Autodesk Inventor part; units mm, degrees
ref_plane "YZ Plane" through (0, 0, 0) normal (1, 0, 0) x (0, 1, 0)
ref_plane "XZ Plane" through (0, 0, 0) normal (0, 1, 0) x (-1, 0, 0)
ref_plane "XY Plane" through (0, 0, 0) normal (0, 0, 1) x (1, 0, 0)
sketch "Sketch1" plane through (0, 0, 0) normal (0, 0, 1) x (1, 0, 0)
  circle A0 centre (0, 0) radius 195 construction
  line L0 (0, 195) -> (0, 225) construction
  line L1 (0, 195) -> (0, 165) construction
  circle A1 centre (0, 0) radius 165
  circle A2 centre (0, 0) radius 225
  line L2 (-165, 0) -> (-165, 80)
  line L3 (-165, 80) -> (-225, 80)
  line L4 (-225, 80) -> (-225, 0)
  line L5 (165, 0) -> (165, 80)
  line L6 (165, 80) -> (225, 80)
  line L7 (225, 80) -> (225, 0)
  line L8 (-225, 0) -> (-165, 0)
  line L9 (165, 0) -> (225, 0)
  line L10 (-225, 0) -> (-285, 0)
  line L11 (-285, 0) -> (-285, -50)
  line L12 (-285, -50) -> (-219.3741, -50)
  line L13 (225, 0) -> (285, 0)
  line L14 (285, 0) -> (285, -50)
  line L15 (285, -50) -> (219.3741, -50)
  dimension "d13" = 390
  dimension "d26" = 80
  dimension "d36" = 60
  dimension "d40" = 60
  dimension "d41" = 50
extrude "Extrusion1" add sketch "Sketch1" against normal blind 30 contours L9 A2 L8 A1 | L13 L14 L15 A2 | A2 L12 L11 L10
sketch "Sketch4" plane through (0, 0, 0) normal (0, 0, 1) x (1, 0, 0)
  circle A0 centre (38.0426, -191.2531) radius 6.5
  line L0 (0, 0) -> (38.0426, -191.2531) construction
  line L1 (0, 0) -> (0, -276.8337) construction
  dimension "d17" = 13
  dimension "d27" = 195
  dimension "d35" = 11.25
extrude "Extrusion4" cut sketch "Sketch4" against normal through all
sketch "Sketch5" plane through (0, 0, 0) normal (0, 0, 1) x (1, 0, 0)
  circle A0 centre (38.0426, -191.2531) radius 6.5
  circle A1 centre (38.0426, -191.2531) radius 17.5
  point P0 (0, 0)
  dimension "d23" = 35
extrude "Extrusion5" cut sketch "Sketch5" against normal blind 15
pattern_circular "Circular Pattern3" count 8 over 157.5 about axis through (0, 0, 0) along (0, 0, -1) of "Extrusion4", "Extrusion5" both ways yes
sketch "Sketch7" plane through (-285, 0, 0) normal (0, 1, 0) x (1, 0, 0)
  circle A0 centre (25, 15) radius 7
  line L0 (0, 0) -> (0, 30)
  point P0 (285, 0)
  point P1 (0, 15)
  dimension "d42" = 14
  dimension "d43" = 25
extrude "Extrusion7" cut sketch "Sketch7" against normal through all
mirror "Mirror1" about plane through (0, 0, 0) normal (1, 0, 0) of "Extrusion7"
equation "\"d13\" = Шпил_пласт_НОС_диам_центров"
equation "\"d40\" = d36"
equation "\"d27\" = 0.5 * Шпил_пласт_НОС_диам_центров"
equation "\"BendReliefDepth\" = 0.5 * Thickness"
properties part number "ДМФ 091 Постель НОС"
Geometry: final body of the model. Coordinates: model frame, mm. A direction names the side the tool comes from. Coordinates: 2 decimals unless noted, no trailing zeros. Order: outer loops, then holes, each group sorted by start corner. A loop starts at its lowest first (then second) coordinate and runs counter-clockwise, first axis right, second up. Notation, with made-up numbers: (58.5, -5) - (78.5, -5) arc R16 cw to (78.5, 11) - close; hole circle Ø3 at (69.25, 4.25). An arc over 180 degrees is marked (long way). Return JSON: item names as keys, results as strings. Group by question number.
1. Cut plane B-B (y = -76). Output: boundary loops of the cut face in (x, z).
2. Cut plane C-C (x = 0). Output: boundary loops of the cut face in (y, z).
3. Cut plane D-D (x = -234.5). Output: boundary loops of the cut face in (y, z).
4. Pull-direction query (Y, two-part tool) for faces 3 (the face through (46, -191, -15)), 4 (the face through (252.6, -50, -14.8)), 5 (the face through (41.04, -197.02, -22.4)), 6 (the face through (-22, -170, -30)); classes: pulls with the +Y half, pulls with the -Y half, needs draft (parallel to the pull), parting line crosses it, or undercut.
5. Pin query (flat end, axial travel): pin 1 (10.5 mm diameter, centred on x = 167, y = -117, fed in from +Z); pin 2 (12 mm diameter, centred on x = 185, z = -9.5, fed in from -Y); pin 3 (1 mm diameter, centred on x = 50, z = -7, fed in from -Y). Return the tip coordinate at first contact, or that it passes through.
6. Material intervals for line 1 along X through (y, z) = (-168, -4.75); line 2 along X through (y, z) = (-120, -6); line 3 along X through (y, z) = (-123, -1.25), sorted ascending. Write a range as [from, to].
7. Set-up query: faces 1 (the face through (-109.093, -144.653, -7.395)), 2 (the face through (224, 0, -15)). Return all of +Z, -Z, +X, -X, +Y, -Y with unobstructed straight access to the full face (end or side cutting, diameter ignored); none if empty.
8. Cut plane A-A (x = 260). Output: boundary loops of the cut face in (y, z), plus the area to 3 significant figures.
Resolved:
{
 "1": {"outline": "(-211.78, -30) - (-146.45, -30) - (-146.45, 0) - (-211.78, 0) - close; (146.45, -30) - (211.78, -30) - (211.78, 0) - (146.45, 0) - close"},
 "2": {"outline": "(-225, -30) - (-165, -30) - (-165, 0) - (-225, 0) - close"},
 "3": {"outline": "(-50, -30) - (0, -30) - (0, 0) - (-50, 0) - close"},
 "4": {"face 3": "undercut", "face 4": "pulls with the -Y half", "face 5": "undercut", "face 6": "needs draft"},
 "5": {"pin 1": "stops at z = -15", "pin 2": "stops at y = -136.32", "pin 3": "stops at y = -219.49"},
 "6": {"line 1": "x = [-149.67, -124.82], [-91.85, 91.85], [124.82, 149.67]", "line 2": "x = [-190.33, -175.18], [-149.09, -113.25], [113.25, 149.09], [175.18, 190.33]", "line 3": "x = [-188.4, -171.69], [-152.59, -109.98], [109.98, 152.59], [171.69, 188.4]"},
 "7": {"face 1": "+Z", "face 2": "+Z, -Z, +X, -X, +Y"},
 "8": {"outline": "(-50, -30) - (0, -30) - (0, -22) - (-50, -22) - close; (-50, -8) - (0, -8) - (0, 0) - (-50, 0) - close", "area": "800 mm²"}
}
